Part model, mm, in its own coordinate system. Face numbers are marked on the shaded views. A direction names the side the tool comes from. Coordinates: 2 decimals unless noted, no trailing zeros. Write each loop counter-clockwise with the first axis right and the second up, starting at its lowest first coordinate (ties: lowest second). Pieces come first, ordered by that corner, then holes. Notation, with made-up numbers: (-11.5, 18) - (4.5, 18) arc R23 cw to (4.5, 36) - close; hole circle Ø7 at (-34.5, 4.5). An arc over 180 degrees is marked (long way). Write each question's results on one line, items separated by ' | '.
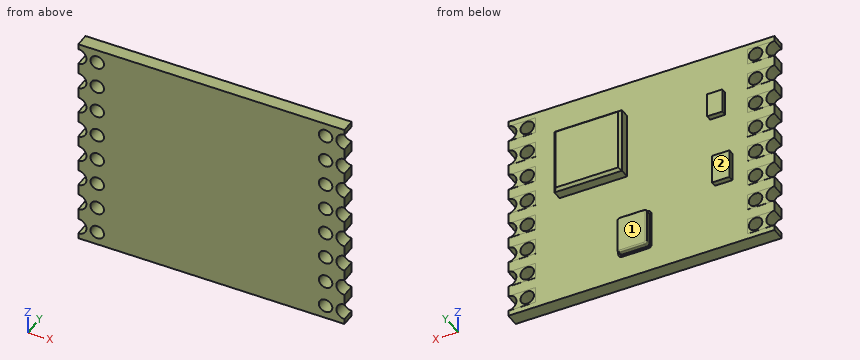
from build123d import *

# Parameters (mm, degrees)
SKETCH1_W           = 19.7
SKETCH1_H           = 16
BOSS_EXTRUDE1_DEPTH = 1
SKETCH2_W           = 2
SKETCH2_H           = 1.2
BOSS_EXTRUDE2_DEPTH = 0.01
SKETCH3_R           = 0.5
CUT_EXTRUDE1_DEPTH  = 1.01
SKETCH4_W           = 5
SKETCH4_H           = 5
BOSS_EXTRUDE3_DEPTH = 0.9
SKETCH5_W           = 1.118442439
SKETCH5_H           = 1.825254878
SKETCH5_W_2         = 1.288131099
SKETCH5_H_2         = 2.193633861
BOSS_EXTRUDE4_DEPTH = 0.4
BOSS_EXTRUDE5_DEPTH = 0.1
BOSS_EXTRUDE6_DEPTH = 0.4
FILLET1_R           = 0.1
CHAMFER1_SIZE       = 0.2


with BuildPart() as part:
    # Sketch1 → Boss-Extrude1 (new body)
    with BuildSketch(Plane(origin=(0, 0, 0), x_dir=(1, 0, 0), z_dir=(0, 1, 0))):
        with Locations((9.85, 8)):
            Rectangle(SKETCH1_W, SKETCH1_H)
    extrude(amount=BOSS_EXTRUDE1_DEPTH)

    # Sketch2 → Boss-Extrude2 (add)
    with BuildSketch(Plane(origin=(0, 1, 0), x_dir=(1, 0, 0), z_dir=(0, 1, 0))):
        with Locations((1, 15)):
            Rectangle(SKETCH2_W, SKETCH2_H)
        with Locations((1, 13)):
            Rectangle(SKETCH2_W, SKETCH2_H)
        with Locations((1, 11)):
            Rectangle(SKETCH2_W, SKETCH2_H)
        with Locations((1, 9)):
            Rectangle(SKETCH2_W, SKETCH2_H)
        with Locations((1, 7)):
            Rectangle(SKETCH2_W, SKETCH2_H)
        with Locations((1, 5)):
            Rectangle(SKETCH2_W, SKETCH2_H)
        with Locations((1, 3)):
            Rectangle(SKETCH2_W, SKETCH2_H)
        with Locations((1, 1)):
            Rectangle(SKETCH2_W, SKETCH2_H)
        with Locations((18.7, 15)):
            Rectangle(SKETCH2_W, SKETCH2_H)
        with Locations((18.7, 13)):
            Rectangle(SKETCH2_W, SKETCH2_H)
        with Locations((18.7, 11)):
            Rectangle(SKETCH2_W, SKETCH2_H)
        with Locations((18.7, 9)):
            Rectangle(SKETCH2_W, SKETCH2_H)
        with Locations((18.7, 7)):
            Rectangle(SKETCH2_W, SKETCH2_H)
        with Locations((18.7, 5)):
            Rectangle(SKETCH2_W, SKETCH2_H)
        with Locations((18.7, 3)):
            Rectangle(SKETCH2_W, SKETCH2_H)
        with Locations((18.7, 1)):
            Rectangle(SKETCH2_W, SKETCH2_H)
    extrude(amount=BOSS_EXTRUDE2_DEPTH)

    # Sketch3 → Cut-Extrude1 (cut)
    with BuildSketch(Plane(origin=(0, 1.01, 0), x_dir=(1, 0, 0), z_dir=(0, 1, 0))):
        with Locations(Location((1.4, 15, 0), (0, 0, 270))):
            Circle(SKETCH3_R)
        with Locations(Location((1.4, 13, 0), (0, 0, 270))):
            Circle(SKETCH3_R)
        with Locations(Location((1.4, 11, 0), (0, 0, 270))):
            Circle(SKETCH3_R)
        with Locations(Location((1.4, 9, 0), (0, 0, 270))):
            Circle(SKETCH3_R)
        with Locations(Location((1.4, 7, 0), (0, 0, 270))):
            Circle(SKETCH3_R)
        with Locations(Location((1.4, 5, 0), (0, 0, 270))):
            Circle(SKETCH3_R)
        with Locations(Location((1.4, 3, 0), (0, 0, 270))):
            Circle(SKETCH3_R)
        with Locations(Location((1.4, 1, 0), (0, 0, 270))):
            Circle(SKETCH3_R)
        with Locations(Location((18.3, 15, 0), (0, 0, 270))):
            Circle(SKETCH3_R)
        with Locations(Location((18.3, 13, 0), (0, 0, 270))):
            Circle(SKETCH3_R)
        with Locations(Location((18.3, 11, 0), (0, 0, 270))):
            Circle(SKETCH3_R)
        with Locations(Location((18.3, 9, 0), (0, 0, 270))):
            Circle(SKETCH3_R)
        with Locations(Location((18.3, 7, 0), (0, 0, 270))):
            Circle(SKETCH3_R)
        with Locations(Location((18.3, 5, 0), (0, 0, 270))):
            Circle(SKETCH3_R)
        with Locations(Location((18.3, 3, 0), (0, 0, 270))):
            Circle(SKETCH3_R)
        with Locations(Location((18.3, 1, 0), (0, 0, 270))):
            Circle(SKETCH3_R)
        with BuildLine():
            Line((0, 15.6), (0, 14.4))
            ThreePointArc((0, 14.4), (0.6, 15), (0, 15.6))
        make_face()
        with BuildLine():
            Line((0, 13.6), (0, 12.4))
            ThreePointArc((0, 12.4), (0.6, 13), (0, 13.6))
        make_face()
        with BuildLine():
            Line((0, 11.6), (0, 10.4))
            ThreePointArc((0, 10.4), (0.6, 11), (0, 11.6))
        make_face()
        with BuildLine():
            Line((0, 9.6), (0, 8.4))
            ThreePointArc((0, 8.4), (0.6, 9), (0, 9.6))
        make_face()
        with BuildLine():
            Line((0, 7.6), (0, 6.4))
            ThreePointArc((0, 6.4), (0.6, 7), (0, 7.6))
        make_face()
        with BuildLine():
            Line((0, 5.6), (0, 4.4))
            ThreePointArc((0, 4.4), (0.6, 5), (0, 5.6))
        make_face()
        with BuildLine():
            Line((0, 3.6), (0, 2.4))
            ThreePointArc((0, 2.4), (0.6, 3), (0, 3.6))
        make_face()
        with BuildLine():
            Line((0, 1.6), (0, 0.4))
            ThreePointArc((0, 0.4), (0.6, 1), (0, 1.6))
        make_face()
        with BuildLine():
            Line((19.7, 15.6), (19.7, 14.4))
            ThreePointArc((19.7, 14.4), (19.1, 15), (19.7, 15.6))
        make_face()
        with BuildLine():
            Line((19.7, 13.6), (19.7, 12.4))
            ThreePointArc((19.7, 12.4), (19.1, 13), (19.7, 13.6))
        make_face()
        with BuildLine():
            Line((19.7, 11.6), (19.7, 10.4))
            ThreePointArc((19.7, 10.4), (19.1, 11), (19.7, 11.6))
        make_face()
        with BuildLine():
            Line((19.7, 9.6), (19.7, 8.4))
            ThreePointArc((19.7, 8.4), (19.1, 9), (19.7, 9.6))
        make_face()
        with BuildLine():
            Line((19.7, 7.6), (19.7, 6.4))
            ThreePointArc((19.7, 6.4), (19.1, 7), (19.7, 7.6))
        make_face()
        with BuildLine():
            Line((19.7, 5.6), (19.7, 4.4))
            ThreePointArc((19.7, 4.4), (19.1, 5), (19.7, 5.6))
        make_face()
        with BuildLine():
            Line((19.7, 3.6), (19.7, 2.4))
            ThreePointArc((19.7, 2.4), (19.1, 3), (19.7, 3.6))
        make_face()
        with BuildLine():
            Line((19.7, 1.6), (19.7, 0.4))
            ThreePointArc((19.7, 0.4), (19.1, 1), (19.7, 1.6))
        make_face()
    extrude(amount=-CUT_EXTRUDE1_DEPTH, mode=Mode.SUBTRACT)

    # Sketch4 → Boss-Extrude3 (add)
    with BuildSketch(Plane(origin=(0, 1, 0), x_dir=(1, 0, 0), z_dir=(0, 1, 0))):
        with Locations((13.417484737, 5.161104769)):
            Rectangle(SKETCH4_W, SKETCH4_H)
    extrude(amount=BOSS_EXTRUDE3_DEPTH)

    # Sketch5 → Boss-Extrude4 (add)
    with BuildSketch(Plane(origin=(0, 1, 0), x_dir=(1, 0, 0), z_dir=(0, 1, 0))):
        with Locations((4.211907739, 4.273374336)):
            Rectangle(SKETCH5_W, SKETCH5_H)
        with Locations((3.772536097, 9.673616078)):
            Rectangle(SKETCH5_W_2, SKETCH5_H_2)
    extrude(amount=BOSS_EXTRUDE4_DEPTH)

    # Sketch6 → Boss-Extrude5 (add)
    with BuildSketch(Plane(origin=(0, 1, 0), x_dir=(1, 0, 0), z_dir=(0, 1, 0))):
        with BuildLine():
            Line((9.314947629, 14.164496182), (11.314947629, 14.164496182))
            ThreePointArc((11.314947629, 14.164496182), (11.456368986, 14.105917538), (11.514947629, 13.964496182))
            Line((11.514947629, 13.964496182), (11.514947629, 11.364496182))
            ThreePointArc((11.514947629, 11.364496182), (11.456368986, 11.223074825), (11.314947629, 11.164496182))
            Line((11.314947629, 11.164496182), (9.314947629, 11.164496182))
            ThreePointArc((9.314947629, 11.164496182), (9.173526273, 11.223074825), (9.114947629, 11.364496182))
            Line((9.114947629, 11.364496182), (9.114947629, 13.964496182))
            ThreePointArc((9.114947629, 13.964496182), (9.173526273, 14.105917538), (9.314947629, 14.164496182))
        make_face()
    extrude(amount=BOSS_EXTRUDE5_DEPTH)

    # Sketch7 → Boss-Extrude6 (add)
    with BuildSketch(Plane(origin=(0, 1.1, 0), x_dir=(1, 0, 0), z_dir=(0, 1, 0))):
        with BuildLine():
            Line((9.414947629, 14.064496182), (11.214947629, 14.064496182))
            ThreePointArc((11.214947629, 14.064496182), (11.356368986, 14.005917538), (11.414947629, 13.864496182))
            Line((11.414947629, 13.864496182), (11.414947629, 11.464496182))
            ThreePointArc((11.414947629, 11.464496182), (11.356368986, 11.323074825), (11.214947629, 11.264496182))
            Line((11.214947629, 11.264496182), (9.414947629, 11.264496182))
            ThreePointArc((9.414947629, 11.264496182), (9.273526273, 11.323074825), (9.214947629, 11.464496182))
            Line((9.214947629, 11.464496182), (9.214947629, 13.864496182))
            ThreePointArc((9.214947629, 13.864496182), (9.273526273, 14.005917538), (9.414947629, 14.064496182))
        make_face()
    extrude(amount=BOSS_EXTRUDE6_DEPTH)

    # Fillet1
    fillet1_edges = [part.edges().sort_by_distance(p)[0] for p in [
        (11.356368986, 1.5, -14.005917538),
        (10.314947629, 1.5, -14.064496182),
        (9.273526273, 1.5, -14.005917538),
        (9.214947629, 1.5, -12.664496182),
        (9.273526273, 1.5, -11.323074825),
        (10.314947629, 1.5, -11.264496182),
        (11.356368986, 1.5, -11.323074825),
        (11.414947629, 1.5, -12.664496182),
    ]]
    fillet(fillet1_edges, radius=FILLET1_R)

    # Chamfer1
    chamfer1_edges = [part.edges().sort_by_distance(p)[0] for p in [
        (10.917484737, 1.9, -5.161104769),
        (13.417484737, 1.9, -2.661104769),
        (15.917484737, 1.9, -5.161104769),
        (13.417484737, 1.9, -7.661104769),
    ]]
    chamfer(chamfer1_edges, length=CHAMFER1_SIZE)


solid = part.part
(1) Flat gauge pins, fed straight in: P1, Ø0.6, axis at y = 1.5, z = -5, coming from the -X side; P2, Ø1, axis at x = 14.5, z = -10.5, coming from the +Y side. Where does each tip first touch, or does it go through?
Return value:
P1: stops at x = 3.65 | P2: stops at y = 1
(2) Saw through at D-D on z = -4. Write the cut outline in (x, y).
Return value:
outline: (0, 0) - (19.7, 0) - (19.7, 1) - (15.92, 1) - (15.92, 1.7) - (15.72, 1.9) - (11.12, 1.9) - (10.92, 1.7) - (10.92, 1) - (4.77, 1) - (4.77, 1.4) - (3.65, 1.4) - (3.65, 1) - (0, 1) - close
(3) Saw through at A-A on z = -13. Count the separate pieces of the cut face and the enclosed holes in it, then the cut area to 3 significant figures.
Return value:
separate pieces: 3 | enclosed holes: 0 | area: 17.6 mm^2
(4) 3-axis set-ups, long thin cutter, end or side, ignore diameter. For the marked faces 1 and 2: which of +Z, -Z, +X, -X, +Y, -Y reach the whole face in a straight line?
Return value:
face 1: -Z, +X, -X, +Y | face 2: +Z, -Z, +X, -X, +Y
(5) Wall check: line 1 (X direction, y = 0.35, z = -11); line 2 (Z direction, x = 4.25, y = 1.25); line 3 (X direction, y = 0.6, z = -7.25). Give the ranges that are in metal, low to high. Write a range as from..to.
Return value:
line 1: x = 0.6..0.9, 1.9..17.8, 18.8..19.1 | line 2: z = -10.77..-8.58, -5.19..-3.36 | line 3: x = 0.55..0.97, 1.83..17.87, 18.73..19.15
